```python
from build123d import *

# Parameters (mm, degrees)
BOSS_EXTRUDE1_DEPTH = 9.525
CUT_EXTRUDE1_START  = -4.445
CUT_EXTRUDE1_DEPTH  = 4.445
SKETCH3_R           = 1.905
SKETCH3_W           = 6.35
SKETCH3_H           = 6.35
CUT_EXTRUDE2_DEPTH  = 252.056346263


with BuildPart() as part:
    # Sketch1 → Boss-Extrude1 (new body)
    with BuildSketch(Plane.XY):
        with BuildLine():
            Line((37.887154169, 1.47019733), (27.071909447, -21.512197706))
            Line((27.071909447, -21.512197706), (33.138342598, -24.366989778))
            Line((33.138342598, -24.366989778), (60.90777145, 41.722489626))
            Line((60.90777145, 41.722489626), (157.204972785, 179.808197732))
            Line((157.204972785, 179.808197732), (157.605048009, 186.145582036))
            ThreePointArc((157.605048009, 186.145582036), (156.833701368, 192.411577396), (151.038083589, 194.915272276))
            Line((151.038083589, 194.915272276), (137.156365398, 193.347216127))
            Line((137.156365398, 193.347216127), (25.899136681, 33.809524518))
            Line((25.899136681, 33.809524518), (0, 0))
            Line((0, 0), (25.00366663, 13.61700957))
            ThreePointArc((25.00366663, 13.61700957), (35.848848557, 12.214099668), (37.887154169, 1.47019733))
        make_face()
    extrude(amount=BOSS_EXTRUDE1_DEPTH)

    # Sketch2 → Cut-Extrude1 (cut)
    with BuildSketch(Plane.XY.offset(9.525).offset(CUT_EXTRUDE1_START)):
        with BuildLine():
            Line((149.320840168, 168.502718236), (145.525755772, 187.35205629))
            ThreePointArc((145.525755772, 187.35205629), (146.619175628, 192.34552843), (151.038083589, 194.915272276))
            ThreePointArc((151.038083589, 194.915272276), (156.833701368, 192.411577396), (157.605048009, 186.145582036))
            Line((157.605048009, 186.145582036), (157.204972785, 179.808197732))
            Line((157.204972785, 179.808197732), (149.320840168, 168.502718236))
        make_face()
    extrude(amount=CUT_EXTRUDE1_DEPTH, mode=Mode.SUBTRACT)

    # Sketch3 → Cut-Extrude2 (cut, through all)
    with BuildSketch(Plane.XY.offset(5.08)):
        with Locations((151.750836383, 180.350400371)):
            Circle(SKETCH3_R)
        with Locations((151.750836383, 188.605400371)):
            Rectangle(SKETCH3_W, SKETCH3_H)
    extrude(amount=-CUT_EXTRUDE2_DEPTH, mode=Mode.SUBTRACT)


solid = part.part
```
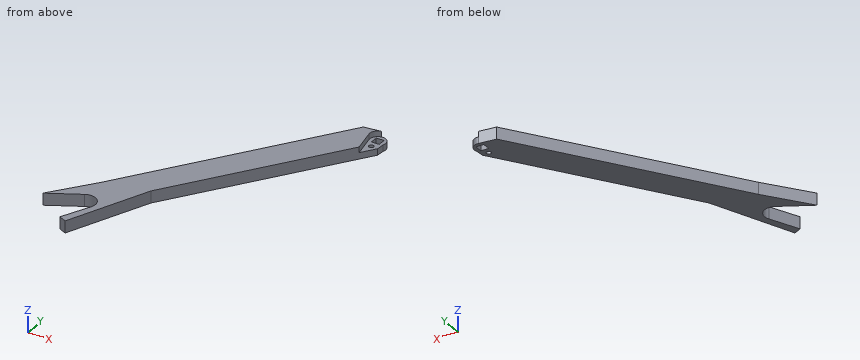
Verification items for the finished model (mm, model axes). Round coordinates to 2 decimals unless told otherwise and drop trailing zeros. Write each loop counter-clockwise with the first axis right and the second up, starting at its lowest first coordinate (ties: lowest second). Pieces come first, ordered by that corner, then holes.
1. Gauge pin test, flat ends, axial feed: P1, Ø1, axis at x = 22.5, z = 7.5, coming from the -Y side; P2, Ø4, axis at y = 23.5, z = 6.5, coming from the +X side; P3, Ø3, axis at x = 51, z = 8, coming from the -Y side. Record the tip position at first contact, or that the pin passes through.
2. Section check A-A on y = 7.5. Enter the section's corners in (x, z) (3 decimals), plus the area to 3 significant figures.
3. Section check B-B on z = 1.5. State how many separate pieces and enclosed holes the cut face has, plus the area to 3 significant figures.
4. Section check C-C on x = 13.5. Enter the section's corners in (y, z) (3 decimals).
5. Scan lines: L1, parallel to X at y = 3.5, z = 4.5; L2, parallel to Y at x = 35.5, z = 6.25; L3, parallel to Y at x = 10, z = 2. Record each from-to range of solid material in increasing order.
6. Section check D-D on y = 142. Enter the section's corners in (x, z) (3 decimals), plus the area to 3 significant figures.
Answer:
1. P1: stops at y = 11.98
1. P2: stops at x = 54.09
1. P3: stops at y = 14.57
2. outline: (5.745, 0) - (13.772, 0) - (13.772, 9.525) - (5.745, 9.525) - close; (38.542, 0) - (46.528, 0) - (46.528, 9.525) - (38.542, 9.525) - close
2. area: 153 mm2
3. separate pieces: 1
3. enclosed holes: 2
3. area: 5,690 mm2
4. outline: (7.352, 0) - (17.623, 0) - (17.623, 9.525) - (7.352, 9.525) - close
5. L1: x = 2.68 to 6.43, 38.57 to 44.85
5. L2: y = -18.75 to -3.6, 12.53 to 47.58
5. L3: y = 5.45 to 13.05
6. outline: (101.348, 0) - (130.839, 0) - (130.839, 9.525) - (101.348, 9.525) - close
6. area: 281 mm2
